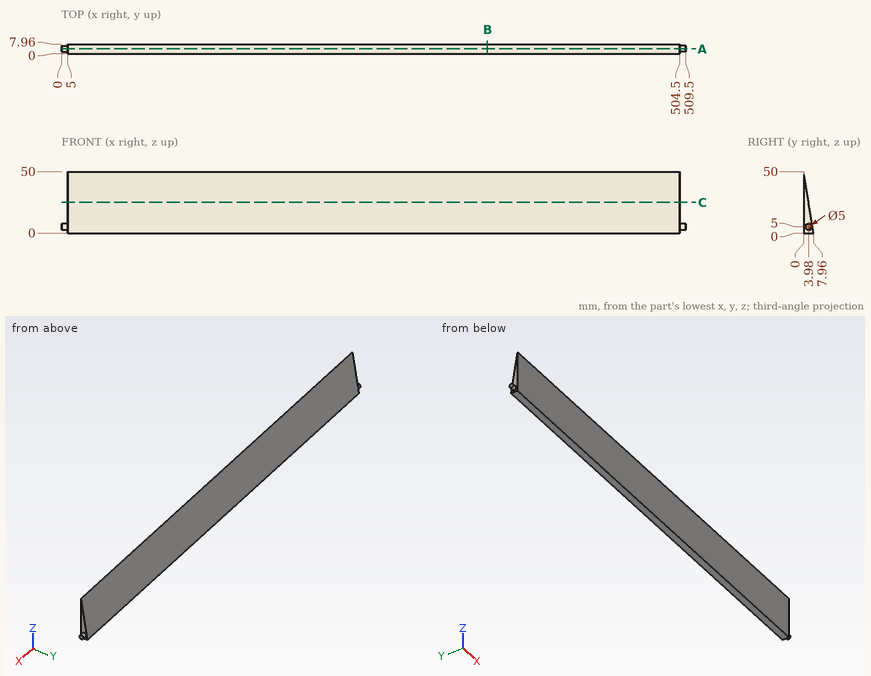
Here's the drawing with two shaded views (mm, measured from the low corner). I have some questions. Give positions to 0.01 mm unless a question says otherwise; leave off trailing zeros. Loops run counter-clockwise (first coordinate to the right, second up) from the corner with the lowest first, then second, coordinate; pieces in that order, holes last. Notation, with made-up numbers: (-38, -38) - (-16, -38) arc R9 cw to (-16, -30) - close; hole circle Ø10 at (62.25, -1.75). An arc over 180 degrees is marked (long way). Answer in a Markdown table with one row per item. Add a question column.
Q1. For pin 1 (6 mm diameter, centred on x = 407.5, z = 11, fed in from +Y); pin 2 (2.5 mm diameter, centred on y = 5.5, z = 35.5, fed in from -X); pin 3 (1 mm diameter, centred on y = 2, z = 18, fed in from -X); pin 4 (4 mm diameter, centred on y = 4.5, z = 32, fed in from +X), each with a flat end and sliding along its axis, tell me the tip position at first contact or that it passes through.
Q2. If we section it at C-C (z = 25): List the corners of the cut face in (x, y) for me, plus the area to 3 significant figures.
Q3. If we section it at B-B (x = 347.5): List the corners of the cut face in (y, z) for me, plus the area to 3 significant figures.
Q4. If we section it at A-A (y = 3.98): List the corners of the cut face in (x, z) for me, plus the area to 3 significant figures.
Q5. Please list where these lines run through material, in increasing order: L1, parallel to X at y = 3, z = 9; L2, parallel to Y at x = 338.5, z = 28.5; L3, parallel to Y at x = 59.5, z = 12. Write a range as from..to.
The answers:
| question | item | result |
|---|---|---|
| 1 | pin 1 | stops at y = 6.69 |
| 1 | pin 2 | passes through |
| 1 | pin 3 | stops at x = 5 |
| 1 | pin 4 | stops at x = 504.5 |
| 2 | outline | (5, 0) - (504.5, 0) - (504.5, 3.98) - (5, 3.98) - close |
| 2 | area | 1,990 mm^2 |
| 3 | outline | (0, 0) - (7.96, 0) - (0, 50) - close |
| 3 | area | 199 mm^2 |
| 4 | outline | (0, 2.5) - (5, 2.5) - (5, 0) - (504.5, 0) - (504.5, 2.5) - (509.5, 2.5) - (509.5, 7.5) - (504.5, 7.5) - (504.5, 25) - (5, 25) - (5, 7.5) - (0, 7.5) - close |
| 4 | area | 12,500 mm^2 |
| 5 | L1 | x = 5..504.5 |
| 5 | L2 | y = 0..3.42 |
| 5 | L3 | y = 0..6.05 |
